Autodesk Inventor part; units mm, degrees
ref_plane "YZ Plane" through (0, 0, 0) normal (1, 0, 0) x (0, 1, 0)
ref_plane "XZ Plane" through (0, 0, 0) normal (0, 1, 0) x (-1, 0, 0)
ref_plane "XY Plane" through (0, 0, 0) normal (0, 0, 1) x (1, 0, 0)
sketch "草圖5" plane through (0, 0, 0) normal (0, 1, 0) x (-1, 0, 0)
  line L0 (7.15, 3) -> (0.85, 3)
  line L1 (0.85, 3) -> (0.85, 0)
  line L2 (0.85, 0) -> (7.15, 0)
  line L3 (7.15, 0) -> (7.15, 3)
  line L4 (0, -0.85) -> (-3, -0.85)
  line L5 (-3, -0.85) -> (-3, -7.15)
  line L6 (-3, -7.15) -> (0, -7.15)
  line L7 (0, -7.15) -> (0, -0.85)
  line L8 (0, 0) -> (25, 0)
  line L9 (25, 0) -> (25, -8)
  line L10 (25, -8) -> (0, -8)
  line L11 (0, -8) -> (0, 0)
  point P0 (7.15, 0)
  dimension "d17" = 0.85
  dimension "d18" = 0.85
  dimension "d19" = 3
  dimension "d20" = 6.3
  dimension "d21" = 6.3
  dimension "d22" = 25
  dimension "d23" = 8
  dimension "d24" = 3
extrude "擠出3" add sketch "草圖5" along normal blind 3
equation "\"d18\" = d17"
equation "\"d20\" = d21"
properties part number "chassis_1_4"
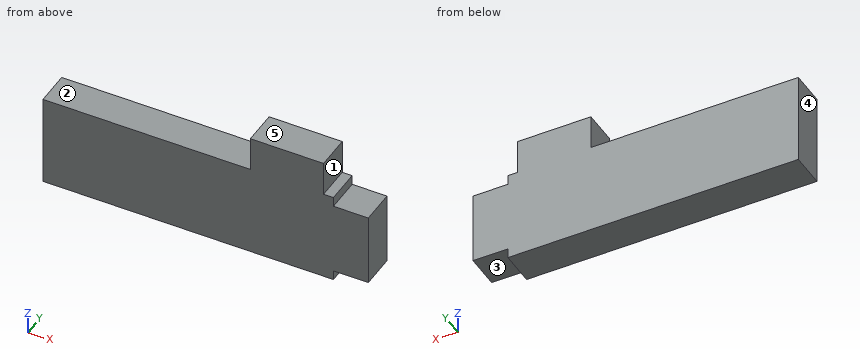
The listing builds one solid part. Answer for the finished solid, in the listing's coordinates (mm). Face numbers are marked on the shaded views. A direction names the side the tool comes from. Give positions to 0.01 mm unless a question says otherwise; leave off trailing zeros. Write each loop counter-clockwise with the first axis right and the second up, starting at its lowest first coordinate (ties: lowest second). Pieces come first, ordered by that corner, then holes. Notation, with made-up numbers: (39.5, 28.5) -> (54.5, 28.5) arc R20 cw to (54.5, 62.5) -> close; hole circle Ø11 at (79, 3). An arc over 180 degrees is marked (long way). Use one line per item in the form item = value.
1) Each of these flat-tipped pins is pushed along its axis until it touches: P1, Ø1.5, axis at x = 1.5, y = 1.5, coming from the +Z side; P2, Ø0.9, axis at x = 1.5, y = 2, coming from the -Z side. Where does it stop, or does it pass through?
Result:
P1 = -0.85
P2 = -7.15
2) Straight lines are drawn through the part: probe 1 along Z at (x, y) = (-19.5, 1.2); probe 2 along X at (y, z) = (0.5, 1.5). For each, find the intervals that lie inside material, in ascending order.
Result:
probe_1 = -8 to 0
probe_2 = -7.15 to -0.85
3) A tool of negligible diameter and unlimited length cuts with its end or side. For the marked faces 1, 2, 3, 4 and 5, from which of +Z, -Z, +X, -X, +Y, -Y can it reach the whole face along a straight path? Write none if from no direction.
Result:
face_1 = +Z, +X, +Y, -Y
face_2 = +Z, -X, +Y, -Y
face_3 = -Z, +X, +Y, -Y
face_4 = +Z, -Z, -X, +Y, -Y
face_5 = +Z, +X, -X, +Y, -Y
4) Section B-B on z = 1.5 is taken. Write down the section's boundary in (x, y), plus the area to 3 significant figures.
Result:
outline = (-7.15, 0) -> (-0.85, 0) -> (-0.85, 3) -> (-7.15, 3) -> close
area = 18.9 mm²
5) Section A-A on y = 2.2 is taken. Write down the section's boundary in (x, z).
Result:
outline = (-25, -8) -> (0, -8) -> (0, -7.15) -> (3, -7.15) -> (3, -0.85) -> (0, -0.85) -> (0, 0) -> (-0.85, 0) -> (-0.85, 3) -> (-7.15, 3) -> (-7.15, 0) -> (-25, 0) -> close
6) Section C-C on x = -21 is taken. Write down the section's boundary in (y, z), plus the area to 3 significant figures.
Result:
outline = (0, -8) -> (3, -8) -> (3, 0) -> (0, 0) -> close
area = 24.0 mm²
